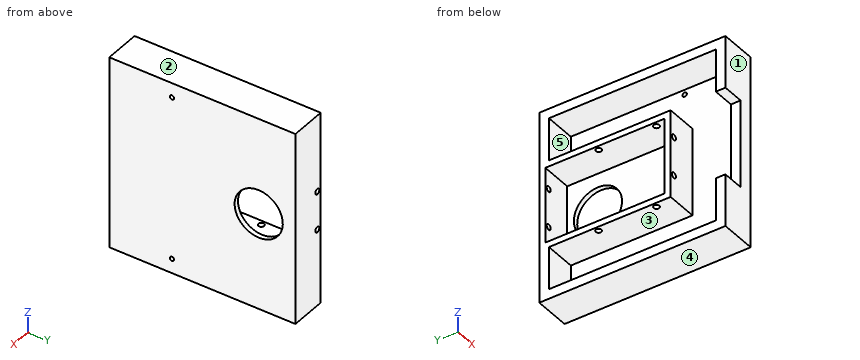
from build123d import *

# Parameters (mm, degrees)
SKETCH_1_W                    = 100
SKETCH_1_H                    = 80
EXTRUDE_1_DEPTH               = 19
SKETCH_2_W                    = 72
SKETCH_2_H                    = 92
CUT_EXTRUDE_1_DEPTH           = 17
SKETCH_3_W                    = 36.5
SKETCH_3_H                    = 54.5
EXTRUDE_2_DEPTH               = 17
SKETCH_4_W                    = 31.5
SKETCH_4_H                    = 49.5
CUT_EXTRUDE_2_DEPTH           = 17
HOLE_WIZARD_20_0_20_1_D       = 20
HOLE_WIZARD_20_0_20_1_DEPTH   = 2
HOLE_WIZARD_2_35_2_35_1_D     = 2.35
HOLE_WIZARD_2_35_2_35_1_DEPTH = 2.5
HOLE_WIZARD_2_35_2_35_2_D     = 2.35
HOLE_WIZARD_2_35_2_35_2_DEPTH = 2.5
HOLE_WIZARD_2_35_2_35_3_D     = 2.35
HOLE_WIZARD_2_35_2_35_3_DEPTH = 2.5
HOLE_WIZARD_2_35_2_35_4_D     = 2.35
HOLE_WIZARD_2_35_2_35_4_DEPTH = 2.5
SKETCH_22_W                   = 13
SKETCH_22_H                   = 36.5
CUT_EXTRUDE_5_DEPTH           = 10
SKETCH_23_W                   = 80
SKETCH_23_H                   = 22.75
CUT_EXTRUDE_6_DEPTH           = 19
SKETCH_24_W                   = 17
SKETCH_24_H                   = 17.75
EXTRUDE_3_DEPTH               = 4
SKETCH_27_W                   = 4
SKETCH_27_H                   = 77.25
CUT_EXTRUDE_7_DEPTH           = 80
SKETCH_28_R                   = 0.9
CUT_EXTRUDE_8_DEPTH           = 10


with BuildPart() as part:
    # 스케치1 → 보스-돌출1 (new body)
    with BuildSketch(Plane(origin=(0, 0, 0), x_dir=(0, -1, 0), z_dir=(-1, 0, 0))):
        with Locations((-23.25, -14.25)):
            Rectangle(SKETCH_1_W, SKETCH_1_H)
    extrude(amount=-EXTRUDE_1_DEPTH)

    # 스케치2 → 컷-돌출1 (cut)
    with BuildSketch(Plane.ZY):
        with Locations((-14.25, 23.25)):
            Rectangle(SKETCH_2_W, SKETCH_2_H)
    extrude(amount=-CUT_EXTRUDE_1_DEPTH, mode=Mode.SUBTRACT)

    # 스케치3 → 보스-돌출2 (add)
    with BuildSketch(Plane.ZY.offset(-17)):
        with Locations((-14.25, 23.25)):
            Rectangle(SKETCH_3_W, SKETCH_3_H)
    extrude(amount=EXTRUDE_2_DEPTH)

    # 스케치4 → 컷-돌출2 (cut)
    with BuildSketch(Plane.ZY):
        with Locations((-14.25, 23.25)):
            Rectangle(SKETCH_4_W, SKETCH_4_H)
    extrude(amount=-CUT_EXTRUDE_2_DEPTH, mode=Mode.SUBTRACT)

    # Ø20.0 (20) 지름 구멍1
    with Locations(Plane.ZY.offset(-17)):
        with Locations((-14.25, 35.25)):
            Hole(HOLE_WIZARD_20_0_20_1_D / 2, depth=HOLE_WIZARD_20_0_20_1_DEPTH)

    # Ø2.35 (2.35) 지름 구멍1
    with Locations(Plane(origin=(0, -1.5, 0), x_dir=(1, 0, 0), z_dir=(0, 1, 0))):
        with Locations((6, 6.25), (6, 22.25)):
            Hole(HOLE_WIZARD_2_35_2_35_1_D / 2, depth=HOLE_WIZARD_2_35_2_35_1_DEPTH)

    # Ø2.35 (2.35) 지름 구멍2
    with Locations(Plane.XY.offset(-30)):
        with Locations((6, 27.25), (6, 3.25)):
            Hole(HOLE_WIZARD_2_35_2_35_2_D / 2, depth=HOLE_WIZARD_2_35_2_35_2_DEPTH)

    # Ø2.35 (2.35) 지름 구멍3
    with Locations(Plane(origin=(0, 48, 0), x_dir=(-1, 0, 0), z_dir=(0, -1, 0))):
        with Locations((-6, 6.25), (-6, 22.25)):
            Hole(HOLE_WIZARD_2_35_2_35_3_D / 2, depth=HOLE_WIZARD_2_35_2_35_3_DEPTH)

    # Ø2.35 (2.35) 지름 구멍4
    with Locations(Plane(origin=(0, 0, 1.5), x_dir=(-1, 0, 0), z_dir=(0, 0, -1))):
        with Locations((-6, 27.25), (-6, 3.25)):
            Hole(HOLE_WIZARD_2_35_2_35_4_D / 2, depth=HOLE_WIZARD_2_35_2_35_4_DEPTH)

    # 스케치22 → 컷-돌출5 (cut)
    with BuildSketch(Plane.XZ.offset(26.75)):
        with Locations((6.5, -14.25)):
            Rectangle(SKETCH_22_W, SKETCH_22_H)
    extrude(amount=-CUT_EXTRUDE_5_DEPTH, mode=Mode.SUBTRACT)

    # 스케치23 → 컷-돌출6 (cut)
    with BuildSketch(Plane.ZY):
        with Locations((-14.25, 61.875)):
            Rectangle(SKETCH_23_W, SKETCH_23_H)
    extrude(amount=-CUT_EXTRUDE_6_DEPTH, mode=Mode.SUBTRACT)

    # 스케치24 → 보스-돌출3 (add)
    with BuildSketch(Plane(origin=(0, 50.5, 0), x_dir=(1, 0, 0), z_dir=(0, 1, 0))):
        with Locations((8.5, -12.875)):
            Rectangle(SKETCH_24_W, SKETCH_24_H)
        with Locations((8.5, 41.375)):
            Rectangle(SKETCH_24_W, SKETCH_24_H)
    extrude(amount=-EXTRUDE_3_DEPTH)

    # 스케치27 → 컷-돌출7 (cut)
    with BuildSketch(Plane(origin=(0, 0, -54.25), x_dir=(-1, 0, 0), z_dir=(0, 0, -1))):
        with Locations((-2, 11.875)):
            Rectangle(SKETCH_27_W, SKETCH_27_H)
    extrude(amount=-CUT_EXTRUDE_7_DEPTH, mode=Mode.SUBTRACT)

    # 스케치28 → 컷-돌출8 (cut)
    with BuildSketch(Plane(origin=(19, 0, 0), x_dir=(0, 0, -1), z_dir=(1, 0, 0))):
        with Locations((-19.725, -0.75)):
            Circle(SKETCH_28_R)
        with Locations((48.225, -0.75)):
            Circle(SKETCH_28_R)
    extrude(amount=-CUT_EXTRUDE_8_DEPTH, mode=Mode.SUBTRACT)


solid = part.part
CAD build for the part. Positions are in the model's coordinates, mm. Face numbers are marked on the shaded views. A direction names the side the tool comes from. Coordinates: 2 decimals unless noted, no trailing zeros. Order: outer loops, then holes, each group sorted by start corner. A loop starts at its lowest first (then second) coordinate and runs counter-clockwise, first axis right, second up.
Item 1: Band-saw the part on A-A on z = -14.25. List the corners of the cut face in (x, y).
Check sheet entries:
outline: (4, -4) - (17, -4) - (17, -22.75) - (13, -22.75) - (13, -26.75) - (19, -26.75) - (19, 25.25) - (17, 25.25) - (17, -1.5) - (4, -1.5) - close; (4, 48) - (17, 48) - (17, 45.25) - (19, 45.25) - (19, 50.5) - (4, 50.5) - close
Item 2: Band-saw the part on B-B on y = 27.25. List the corners of the cut face in (x, z) (3 decimals), plus the area to 3 significant figures.
Check sheet entries:
outline: (4, -54.25) - (19, -54.25) - (19, -20.25) - (17, -20.25) - (17, -30) - (7.175, -30) - (7.175, -32.5) - (17, -32.5) - (17, -50.25) - (4, -50.25) - close; (4, -32.5) - (4.825, -32.5) - (4.825, -30) - (4, -30) - close; (4, 1.5) - (4.825, 1.5) - (4.825, 4) - (4, 4) - close; (4, 21.75) - (17, 21.75) - (17, 4) - (7.175, 4) - (7.175, 1.5) - (17, 1.5) - (17, -8.25) - (19, -8.25) - (19, 25.75) - (4, 25.75) - close
area: 293 mm2
Item 3: Pin check, flat tips, straight feed: pin 1 Ø16 at (y, z) = (26, -10) entering from -X; pin 2 Ø2.5 at (x, z) = (6, -6.25) entering from -Y; pin 3 Ø1.9 at (x, z) = (6, -22.25) entering from +Y. Stop position of each tip, or through.
Check sheet entries:
pin 1: stops at x = 17
pin 2: stops at y = -4
pin 3: passes through
Item 4: 3-axis set-ups, long thin cutter, end or side, ignore diameter. For the marked faces 4 and 5: which of +Z, -Z, +X, -X, +Y, -Y reach the whole face in a straight line?
Check sheet entries:
face 4: -Z, +X, -X, +Y, -Y
face 5: -X
Item 5: Two-plate mould, pull along Z, no slides. Class the marked faces 1, 2 and 3: +Z half, -Z half, draft (parallel to the pull), parting line (faces both ways), or undercut.
Check sheet entries:
face 1: draft
face 2: +Z half
face 3: undercut
Item 6: Band-saw the part on D-D on y = 35.25. List the corners of the cut face in (x, z), plus the area to 3 significant figures.
Check sheet entries:
outline: (4, -54.25) - (19, -54.25) - (19, -24.25) - (17, -24.25) - (17, -30) - (4, -30) - (4, -32.5) - (17, -32.5) - (17, -50.25) - (4, -50.25) - close; (4, 1.5) - (17, 1.5) - (17, -4.25) - (19, -4.25) - (19, 25.75) - (4, 25.75) - (4, 21.75) - (17, 21.75) - (17, 4) - (4, 4) - close
area: 289 mm2
Item 7: Drill centre lines: L1, parallel to Z at x = 13.5, y = 14.5; L2, parallel to Y at x = 15.75, z = 0; L3, parallel to Z at x = 12.75, y = -22. Where is each one in solid material? Low to high.
Check sheet entries:
L1: z = -54.25 to -50.25, -32.5 to -30, 1.5 to 4, 21.75 to 25.75
L2: y = -26.75 to -22.75, -4 to -1.5, 48 to 50.5
L3: z = -54.25 to -50.25, 21.75 to 25.75
Item 8: Band-saw the part on C-C on x = 10.75. List the corners of the cut face in (y, z).
Check sheet entries:
outline: (-26.75, -54.25) - (50.5, -54.25) - (50.5, 25.75) - (-26.75, 25.75) - (-26.75, 4) - (-22.75, 4) - (-22.75, 21.75) - (46.5, 21.75) - (46.5, 4) - (-4, 4) - (-4, -32.5) - (46.5, -32.5) - (46.5, -50.25) - (-22.75, -50.25) - (-22.75, -32.5) - (-26.75, -32.5) - close; hole (-1.5, -30) - (48, -30) - (48, 1.5) - (-1.5, 1.5) - close
